Print and shaded views of the part. All mm, measured from the part's lowest x, y and z. A direction names the side the tool comes from. Give positions to 0.01 mm unless a question says otherwise; leave off trailing zeros. Loops run counter-clockwise (first coordinate to the right, second up) from the corner with the lowest first, then second, coordinate; pieces in that order, holes last. Notation, with made-up numbers: (63.5, 80.25) - (80.5, 80.25) arc R14 ccw to (80.5, 104.25) - close; hole circle Ø8 at (-17.5, 25). An arc over 180 degrees is marked (long way). Return JSON: item names as keys, results as strings.
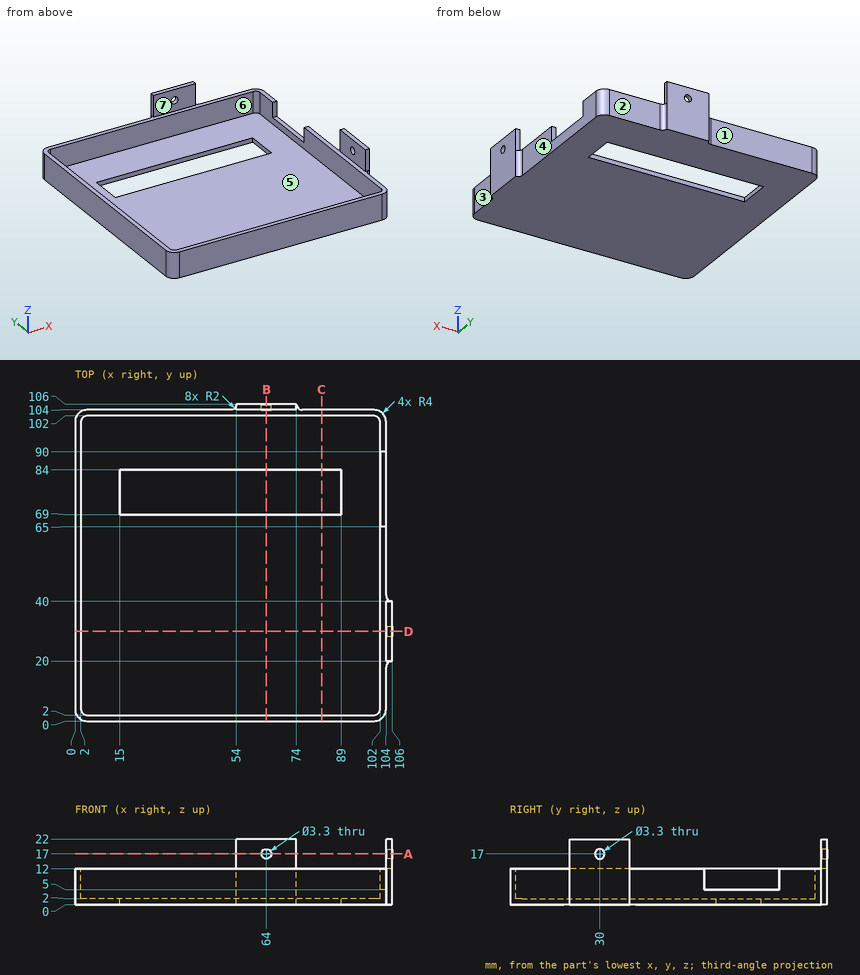
1. Which spindle directions (+Z, -Z, +X, -X, +Y, -Y) get a long thin tool onto all of the face, cutting with end or side? Do the marked faces 1, 2 and 3. Say none if no direction does.
Values follow:
{"face 1": "+Z, -Z, -X, +Y", "face 2": "+Z, -Z, +X, +Y", "face 3": "+Z, -Z, +X, -Y"}
2. Cut at B-B, the plane x = 64. Write the cut outline in (y, z).
Values follow:
{"outline": "(0, 0) - (69, 0) - (69, 2) - (2, 2) - (2, 12) - (0, 12) - close; (84, 0) - (106, 0) - (106, 15.35) - (104, 15.35) - (104, 12) - (102, 12) - (102, 2) - (84, 2) - close; (104, 18.65) - (106, 18.65) - (106, 22) - (104, 22) - close"}
3. Drop flat-ended pins along their axis: P1, Ø8, axis at x = 43.5, y = 82, coming from the +Z side; P2, Ø3, axis at y = 26.5, z = 18.5, coming from the -X side; P3, Ø2, axis at y = 105, z = 16.5, coming from the -X side. Give the stop position or say it passes through.
Values follow:
{"P1": "stops at z = 2", "P2": "stops at x = 104", "P3": "stops at x = 54"}
4. Cut at A-A, the plane z = 17. Write the cut outline in (x, y), plus the area to 3 significant figures.
Values follow:
{"outline": "(54, 104) - (62.35, 104) - (62.35, 106) - (54, 106) - close; (65.65, 104) - (74, 104) - (74, 106) - (65.65, 106) - close; (104, 20) - (106, 20) - (106, 28.35) - (104, 28.35) - close; (104, 31.65) - (106, 31.65) - (106, 40) - (104, 40) - close", "area": "66.8 mm²"}
5. Cut at C-C, the plane x = 82.5. Write the cut outline in (y, z).
Values follow:
{"outline": "(0, 0) - (69, 0) - (69, 2) - (2, 2) - (2, 12) - (0, 12) - close; (84, 0) - (104, 0) - (104, 12) - (102, 12) - (102, 2) - (84, 2) - close"}
6. Drill centre lines: probe 1 along Y at (x, z) = (22.5, 2.75); probe 2 along X at (y, z) = (104.5, 17). Where is each one in solid material? Low to high.
Values follow:
{"probe 1": "y = 0 to 2, 102 to 104", "probe 2": "x = 54 to 62.35, 65.65 to 74"}
7. Pull direction Y, two halves, no side cores. Call the marked faces 4, 5, 6 and 7: +Y half, -Y half, draft (parallel to the pull), parting line (faces both ways), or undercut.
Values follow:
{"face 4": "draft", "face 5": "undercut", "face 6": "undercut", "face 7": "-Y half"}
8. Cut at D-D, the plane y = 30. Write the cut outline in (x, z).
Values follow:
{"outline": "(0, 0) - (106, 0) - (106, 15.35) - (104, 15.35) - (104, 12) - (102, 12) - (102, 2) - (2, 2) - (2, 12) - (0, 12) - close; (104, 18.65) - (106, 18.65) - (106, 22) - (104, 22) - close"}
